Geometry: final body of the model. Coordinates: model frame, mm. A direction names the side the tool comes from. Give positions to 0.01 mm unless a question says otherwise; leave off trailing zeros. Order: outer loops, then holes, each group sorted by start corner. A loop starts at its lowest first (then second) coordinate and runs counter-clockwise, first axis right, second up. Notation, with made-up numbers: M 70,57.25 L 88,57.25 A20 ccw 88,77.25 Z; hole C 28,71.5 d1. An arc over 180 degrees is marked long. One line per item, written item: value. Start each with the question number.
```python
from build123d import *

# Parameters (mm, degrees)
ESBO_O1_W                = 20
ESBO_O1_H                = 430
RESSALTO_EXTRUS_O1_DEPTH = 205
ESBO_O1_3_W              = 390
ESBO_O1_3_H              = 430
ESBO_O1_3_W_2            = 10
RESSALTO_EXTRUS_O2_DEPTH = 30
ESBO_O2_W                = 20
ESBO_O2_H                = 430
RESSALTO_EXTRUS_O4_DEPTH = 30
ESBO_O4_W                = 20
ESBO_O4_H                = 165
CORTE_EXTRUS_O1_DEPTH    = 205
ESBO_O6_R                = 2.5
CORTE_EXTRUS_O3_DEPTH    = 10
RESSALTO_EXTRUS_O6_START = -235
ESBO_O7_W                = 10
ESBO_O7_H                = 100
RESSALTO_EXTRUS_O6_DEPTH = 295
CORTE_EXTRUS_O4_REACH    = 665.344
ESBO_O8_R                = 4
ESBO_O8_R_2              = 1.25
ESBO_O8_R_3              = 1.5
CORTE_EXTRUS_O5_REACH    = 671.571
ESBO_O9_W                = 20
ESBO_O9_H                = 20
CORTE_EXTRUS_O8_REACH    = 671.571
ESBO_O10_R               = 4


with BuildPart() as part:
    # Esbo_o1 → Ressalto-extrus_o1 (new body)
    with BuildSketch(Plane(origin=(0, 0, 0), x_dir=(1, 0, 0), z_dir=(0, 1, 0))):
        with Locations((10, 215)):
            Rectangle(ESBO_O1_W, ESBO_O1_H)
    ressalto_extrus_o1 = extrude(amount=RESSALTO_EXTRUS_O1_DEPTH)

    # Esbo_o1_3 → Ressalto-extrus_o2 (add)
    with BuildSketch(Plane(origin=(0, 0, 0), x_dir=(1, 0, 0), z_dir=(0, 1, 0))):
        with Locations((215, 215)):
            Rectangle(ESBO_O1_3_W, ESBO_O1_3_H)
        with Locations((-5, 215)):
            Rectangle(ESBO_O1_3_W_2, ESBO_O1_3_H)
    ressalto_extrus_o2 = extrude(amount=RESSALTO_EXTRUS_O2_DEPTH)

    # Esbo_o2 → Ressalto-extrus_o4 (add)
    with BuildSketch(Plane(origin=(0, 205, 0), x_dir=(1, 0, 0), z_dir=(0, 1, 0))):
        with Locations((10, 215)):
            Rectangle(ESBO_O2_W, ESBO_O2_H)
    ressalto_extrus_o4 = extrude(amount=RESSALTO_EXTRUS_O4_DEPTH)

    # Esbo_o4 → Corte-extrus_o1 (cut)
    with BuildSketch(Plane(origin=(0, 235, 0), x_dir=(1, 0, 0), z_dir=(0, 1, 0))):
        with Locations((10, 347.5)):
            Rectangle(ESBO_O4_W, ESBO_O4_H)
        with Locations((10, 82.5)):
            Rectangle(ESBO_O4_W, ESBO_O4_H)
    corte_extrus_o1 = extrude(amount=-CORTE_EXTRUS_O1_DEPTH, mode=Mode.SUBTRACT)

    # Esbo_o6 → Corte-extrus_o3 (cut)
    with BuildSketch(Plane(origin=(0, 235, 0), x_dir=(1, 0, 0), z_dir=(0, 1, 0))):
        with Locations(Location((10, 236, 0), (0, 0, 270))):
            Circle(ESBO_O6_R)
        with Locations(Location((10, 194, 0), (0, 0, 270))):
            Circle(ESBO_O6_R)
    corte_extrus_o3 = extrude(amount=-CORTE_EXTRUS_O3_DEPTH, mode=Mode.SUBTRACT)

    # Esbo_o7 → Ressalto-extrus_o6 (add)
    with BuildSketch(Plane(origin=(0, 235, 0), x_dir=(1, 0, 0), z_dir=(0, 1, 0)).offset(RESSALTO_EXTRUS_O6_START)):
        with Locations((-5, 215)):
            Rectangle(ESBO_O7_W, ESBO_O7_H)
    ressalto_extrus_o6 = extrude(amount=RESSALTO_EXTRUS_O6_DEPTH)

    # Esbo_o8 → Corte-extrus_o4 (cut, up to next)
    with BuildSketch(Plane(origin=(0, 0, 0), x_dir=(0, 0, -1), z_dir=(1, 0, 0)), mode=Mode.PRIVATE) as corte_extrus_o4_sk1:
        with Locations((215, 250)):
            Circle(ESBO_O8_R)
    corte_extrus_o4_tool1 = extrude(corte_extrus_o4_sk1.sketch, amount=-CORTE_EXTRUS_O4_REACH, mode=Mode.PRIVATE) & part.part
    # Esbo_o8 → Corte-extrus_o4 (cut, up to next)
    with BuildSketch(Plane(origin=(0, 0, 0), x_dir=(0, 0, -1), z_dir=(1, 0, 0)), mode=Mode.PRIVATE) as corte_extrus_o4_sk2:
        with Locations((205.47, 250)):
            Circle(ESBO_O8_R_2)
    corte_extrus_o4_tool2 = extrude(corte_extrus_o4_sk2.sketch, amount=-CORTE_EXTRUS_O4_REACH, mode=Mode.PRIVATE) & part.part
    # Esbo_o8 → Corte-extrus_o4 (cut, up to next)
    with BuildSketch(Plane(origin=(0, 0, 0), x_dir=(0, 0, -1), z_dir=(1, 0, 0)), mode=Mode.PRIVATE) as corte_extrus_o4_sk3:
        with Locations((224.53, 250)):
            Circle(ESBO_O8_R_2)
    corte_extrus_o4_tool3 = extrude(corte_extrus_o4_sk3.sketch, amount=-CORTE_EXTRUS_O4_REACH, mode=Mode.PRIVATE) & part.part
    # Esbo_o8 → Corte-extrus_o4 (cut, up to next)
    with BuildSketch(Plane(origin=(0, 0, 0), x_dir=(0, 0, -1), z_dir=(1, 0, 0)), mode=Mode.PRIVATE) as corte_extrus_o4_sk4:
        with Locations((215, 259)):
            Circle(ESBO_O8_R_3)
    corte_extrus_o4_tool4 = extrude(corte_extrus_o4_sk4.sketch, amount=-CORTE_EXTRUS_O4_REACH, mode=Mode.PRIVATE) & part.part
    # Esbo_o8 → Corte-extrus_o4 (cut, up to next)
    with BuildSketch(Plane(origin=(0, 0, 0), x_dir=(0, 0, -1), z_dir=(1, 0, 0)), mode=Mode.PRIVATE) as corte_extrus_o4_sk5:
        with Locations((207.205771366, 245.5)):
            Circle(ESBO_O8_R_3)
    corte_extrus_o4_tool5 = extrude(corte_extrus_o4_sk5.sketch, amount=-CORTE_EXTRUS_O4_REACH, mode=Mode.PRIVATE) & part.part
    # Esbo_o8 → Corte-extrus_o4 (cut, up to next)
    with BuildSketch(Plane(origin=(0, 0, 0), x_dir=(0, 0, -1), z_dir=(1, 0, 0)), mode=Mode.PRIVATE) as corte_extrus_o4_sk6:
        with Locations((222.794228634, 245.5)):
            Circle(ESBO_O8_R_3)
    corte_extrus_o4_tool6 = extrude(corte_extrus_o4_sk6.sketch, amount=-CORTE_EXTRUS_O4_REACH, mode=Mode.PRIVATE) & part.part
    corte_extrus_o4_1 = corte_extrus_o4_tool1.solids().sort_by_distance((0, 250, -215))[0]
    add(corte_extrus_o4_1, mode=Mode.SUBTRACT)
    corte_extrus_o4_2 = corte_extrus_o4_tool2.solids().sort_by_distance((0, 250, -205.47))[0]
    add(corte_extrus_o4_2, mode=Mode.SUBTRACT)
    corte_extrus_o4_3 = corte_extrus_o4_tool3.solids().sort_by_distance((0, 250, -224.53))[0]
    add(corte_extrus_o4_3, mode=Mode.SUBTRACT)
    corte_extrus_o4_4 = corte_extrus_o4_tool4.solids().sort_by_distance((0, 259, -215))[0]
    add(corte_extrus_o4_4, mode=Mode.SUBTRACT)
    corte_extrus_o4_5 = corte_extrus_o4_tool5.solids().sort_by_distance((0, 245.5, -207.205771))[0]
    add(corte_extrus_o4_5, mode=Mode.SUBTRACT)
    corte_extrus_o4_6 = corte_extrus_o4_tool6.solids().sort_by_distance((0, 245.5, -222.794229))[0]
    add(corte_extrus_o4_6, mode=Mode.SUBTRACT)
    corte_extrus_o4 = corte_extrus_o4_1 + corte_extrus_o4_2 + corte_extrus_o4_3 + corte_extrus_o4_4 + corte_extrus_o4_5 + corte_extrus_o4_6  # Corte-extrus_o4 as one shape, for the pattern or mirror that repeats it

    # Esbo_o9 → Corte-extrus_o5 (cut, up to next)
    with BuildSketch(Plane.ZY.offset(10), mode=Mode.PRIVATE) as corte_extrus_o5_sk1:
        with Locations((-235, 215)):
            Rectangle(ESBO_O9_W, ESBO_O9_H)
    corte_extrus_o5_tool1 = extrude(corte_extrus_o5_sk1.sketch, amount=-CORTE_EXTRUS_O5_REACH, mode=Mode.PRIVATE) & part.part
    # Esbo_o9 → Corte-extrus_o5 (cut, up to next)
    with BuildSketch(Plane.ZY.offset(10), mode=Mode.PRIVATE) as corte_extrus_o5_sk2:
        with Locations((-195, 215)):
            Rectangle(ESBO_O9_W, ESBO_O9_H)
    corte_extrus_o5_tool2 = extrude(corte_extrus_o5_sk2.sketch, amount=-CORTE_EXTRUS_O5_REACH, mode=Mode.PRIVATE) & part.part
    corte_extrus_o5_1 = corte_extrus_o5_tool1.solids().sort_by_distance((-10, 215, -235))[0]
    add(corte_extrus_o5_1, mode=Mode.SUBTRACT)
    corte_extrus_o5_2 = corte_extrus_o5_tool2.solids().sort_by_distance((-10, 215, -195))[0]
    add(corte_extrus_o5_2, mode=Mode.SUBTRACT)
    corte_extrus_o5 = corte_extrus_o5_1 + corte_extrus_o5_2  # Corte-extrus_o5 as one shape, for the pattern or mirror that repeats it

    # Espelhar1: Ressalto-extrus_o1, Ressalto-extrus_o2, Ressalto-extrus_o4, Corte-extrus_o1, Corte-extrus_o3, Ressalto-extrus_o6, Corte-extrus_o4, Corte-extrus_o5 across plane
    add(ressalto_extrus_o1.mirror(Plane(origin=(205, 0, 0), x_dir=(0, 0, 1), z_dir=(1, 0, 0))))
    add(ressalto_extrus_o2.mirror(Plane(origin=(205, 0, 0), x_dir=(0, 0, 1), z_dir=(1, 0, 0))))
    add(ressalto_extrus_o4.mirror(Plane(origin=(205, 0, 0), x_dir=(0, 0, 1), z_dir=(1, 0, 0))))
    add(corte_extrus_o1.mirror(Plane(origin=(205, 0, 0), x_dir=(0, 0, 1), z_dir=(1, 0, 0))), mode=Mode.SUBTRACT)
    add(corte_extrus_o3.mirror(Plane(origin=(205, 0, 0), x_dir=(0, 0, 1), z_dir=(1, 0, 0))), mode=Mode.SUBTRACT)
    add(ressalto_extrus_o6.mirror(Plane(origin=(205, 0, 0), x_dir=(0, 0, 1), z_dir=(1, 0, 0))))
    add(corte_extrus_o4.mirror(Plane(origin=(205, 0, 0), x_dir=(0, 0, 1), z_dir=(1, 0, 0))), mode=Mode.SUBTRACT)
    add(corte_extrus_o5.mirror(Plane(origin=(205, 0, 0), x_dir=(0, 0, 1), z_dir=(1, 0, 0))), mode=Mode.SUBTRACT)

    # Esbo_o10 → Corte-extrus_o8 (cut, up to next)
    with BuildSketch(Plane(origin=(0, 0, 0), x_dir=(-1, 0, 0), z_dir=(0, -1, 0)), mode=Mode.PRIVATE) as corte_extrus_o8_sk1:
        with Locations(Location((-50, 380, 0), (0, 0, 90))):
            Circle(ESBO_O10_R)
    corte_extrus_o8_tool1 = extrude(corte_extrus_o8_sk1.sketch, amount=-CORTE_EXTRUS_O8_REACH, mode=Mode.PRIVATE) & part.part
    # Esbo_o10 → Corte-extrus_o8 (cut, up to next)
    with BuildSketch(Plane(origin=(0, 0, 0), x_dir=(-1, 0, 0), z_dir=(0, -1, 0)), mode=Mode.PRIVATE) as corte_extrus_o8_sk2:
        with Locations(Location((-50, 50, 0), (0, 0, 90))):
            Circle(ESBO_O10_R)
    corte_extrus_o8_tool2 = extrude(corte_extrus_o8_sk2.sketch, amount=-CORTE_EXTRUS_O8_REACH, mode=Mode.PRIVATE) & part.part
    # Esbo_o10 → Corte-extrus_o8 (cut, up to next)
    with BuildSketch(Plane(origin=(0, 0, 0), x_dir=(-1, 0, 0), z_dir=(0, -1, 0)), mode=Mode.PRIVATE) as corte_extrus_o8_sk3:
        with Locations(Location((-370, 50, 0), (0, 0, 90))):
            Circle(ESBO_O10_R)
    corte_extrus_o8_tool3 = extrude(corte_extrus_o8_sk3.sketch, amount=-CORTE_EXTRUS_O8_REACH, mode=Mode.PRIVATE) & part.part
    # Esbo_o10 → Corte-extrus_o8 (cut, up to next)
    with BuildSketch(Plane(origin=(0, 0, 0), x_dir=(-1, 0, 0), z_dir=(0, -1, 0)), mode=Mode.PRIVATE) as corte_extrus_o8_sk4:
        with Locations(Location((-370, 380, 0), (0, 0, 90))):
            Circle(ESBO_O10_R)
    corte_extrus_o8_tool4 = extrude(corte_extrus_o8_sk4.sketch, amount=-CORTE_EXTRUS_O8_REACH, mode=Mode.PRIVATE) & part.part
    add(corte_extrus_o8_tool1.solids().sort_by_distance((50, 0, -380))[0], mode=Mode.SUBTRACT)
    add(corte_extrus_o8_tool2.solids().sort_by_distance((50, 0, -50))[0], mode=Mode.SUBTRACT)
    add(corte_extrus_o8_tool3.solids().sort_by_distance((370, 0, -50))[0], mode=Mode.SUBTRACT)
    add(corte_extrus_o8_tool4.solids().sort_by_distance((370, 0, -380))[0], mode=Mode.SUBTRACT)


solid = part.part
```
Q1. Section query B-B on z = -252.5. Return loops of the section in (x, y), and give its area (3 significant figures).
Q2. Section query C-C on x = 333.5. Return loops of the section in (y, z), and give its area (3 significant figures).
Q3. Section query D-D on z = -339. Return loops of the section in (x, y), and give its area (3 significant figures).
Q4. Set-up query: faces 4 (the face through (20, 131, -214)), 5 (the face through (208, 0, -218)), 6 (the face through (5, 205, -195)). Return all of +Z, -Z, +X, -X, +Y, -Y with unobstructed straight access to the full face (end or side cutting, diameter ignored); none if empty.
Q5. Section query A-A on y = 166. Return loops of the section in (x, z).
Q6. Contact query for flat-ended pins moving along their axis: pin 1 (1.5 mm diameter, centred on y = 250, z = -224.53, fed in from -X); pin 2 (6 mm diameter, centred on x = 400, y = 215, fed in from -Z); pin 3 (16 mm diameter, centred on x = 5.5, y = 212, fed in from +Z); pin 4 (3 mm diameter, centred on x = 10, z = -194, fed in from +Y). Output: stop coordinate, or through.
Q7. Ray query, line 1 along X through (y, z) = (134, -256); line 2 along Y through (x, z) = (199, -161.5); line 3 along X through (y, z) = (280, -186). Return the intervals inside material, ascending. Write a range as [from, to].
Q8. Mould query, pull axis Z, two halves, no side actions, for faces 1 (the face through (405, 131, -165)), 2 (the face through (405, 205, -235)), 3 (the face through (0, 265, -214)). Classes: +Z half, -Z half, draft (parallel to the pull), parting line (faces both ways), or undercut.
Results below:
1. outline: M -10,0 L 420,0 L 420,295 L 410,295 L 410,235 L 390,235 L 390,30 L 20,30 L 20,235 L 0,235 L 0,295 L -10,295 Z
1. area: 26,400 mm2
2. outline: M 0,-430 L 30,-430 L 30,0 L 0,0 Z
2. area: 12,900 mm2
3. outline: M -10,0 L 420,0 L 420,30 L -10,30 Z
3. area: 12,900 mm2
4. face 4: +Z, -Z, +Y
4. face 5: +Z, -Z, +X, -X, -Y
4. face 6: +X, -X
5. outline: M -10,-265 L 20,-265 L 20,-165 L -10,-165 Z; M 390,-265 L 420,-265 L 420,-165 L 390,-165 Z
6. pin 1: through
6. pin 2: z = -265
6. pin 3: z = -165
6. pin 4: y = 205
7. line 1: [-10, 20], [390, 420]
7. line 2: [0, 30]
7. line 3: [-10, 0], [410, 420]
8. face 1: +Z half
8. face 2: undercut
8. face 3: draft
